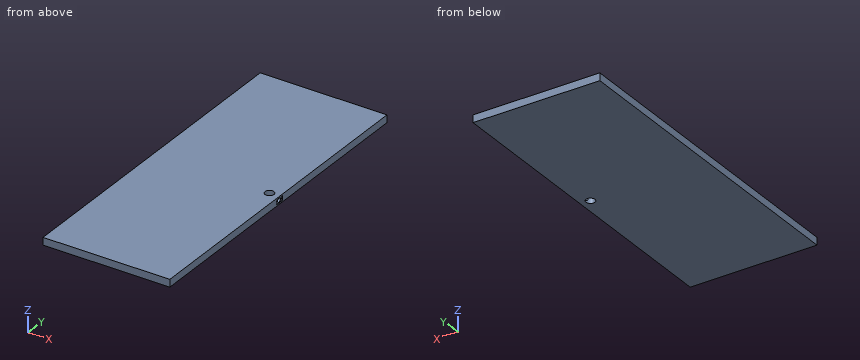
from build123d import *

# Parameters (mm, degrees)
SKETCH1_W           = 765
SKETCH1_H           = 1981
BOSS_EXTRUDE1_DEPTH = 45
SKETCH2_R           = 27
CUT_EXTRUDE1_DEPTH  = 46
CUT_EXTRUDE2_REACH  = 767
SKETCH3_R           = 12.5
SKETCH4_W           = 28.5
SKETCH4_H           = 57
CUT_EXTRUDE3_DEPTH  = 3
SKETCH5_R           = 1.5
CUT_EXTRUDE4_DEPTH  = 15


with BuildPart() as part:
    # Sketch1 → Boss-Extrude1 (new body)
    with BuildSketch(Plane.XY):
        with Locations((382.5, 990.5)):
            Rectangle(SKETCH1_W, SKETCH1_H)
    extrude(amount=BOSS_EXTRUDE1_DEPTH)

    # Sketch2 → Cut-Extrude1 (cut, through all)
    with BuildSketch(Plane.XY.offset(45)):
        with Locations((705, 1000)):
            Circle(SKETCH2_R)
    extrude(amount=-CUT_EXTRUDE1_DEPTH, mode=Mode.SUBTRACT)

    # Sketch3 → Cut-Extrude2 (cut, up to next)
    with BuildSketch(Plane(origin=(765, 0, 0), x_dir=(0, 0, -1), z_dir=(1, 0, 0)), mode=Mode.PRIVATE) as cut_extrude2_sk1:
        with Locations((-22.5, 1000)):
            Circle(SKETCH3_R)
    cut_extrude2_tool1 = extrude(cut_extrude2_sk1.sketch, amount=-CUT_EXTRUDE2_REACH, mode=Mode.PRIVATE) & part.part
    add(cut_extrude2_tool1.solids().sort_by_distance((765, 1000, 22.5))[0], mode=Mode.SUBTRACT)

    # Sketch4 → Cut-Extrude3 (cut)
    with BuildSketch(Plane(origin=(765, 0, 0), x_dir=(0, 0, -1), z_dir=(1, 0, 0))):
        with Locations((-22.5, 1000)):
            Rectangle(SKETCH4_W, SKETCH4_H)
    extrude(amount=-CUT_EXTRUDE3_DEPTH, mode=Mode.SUBTRACT)

    # Sketch5 → Cut-Extrude4 (cut)
    with BuildSketch(Plane(origin=(762, 0, 0), x_dir=(0, 0, -1), z_dir=(1, 0, 0))):
        with Locations((-22.5, 1020.5)):
            Circle(SKETCH5_R)
        with Locations((-22.5, 979.5)):
            Circle(SKETCH5_R)
    extrude(amount=-CUT_EXTRUDE4_DEPTH, mode=Mode.SUBTRACT)


solid = part.part
Build history of the part. All positions in model axes, mm. Give positions to 0.01 mm unless a question says otherwise; leave off trailing zeros. Loops run counter-clockwise (first coordinate to the right, second up) from the corner with the lowest first, then second, coordinate; pieces in that order, holes last. Notation, with made-up numbers: (41, 22) -> (91, 22) arc R32 ccw to (91, 59) -> close; hole circle Ø2 at (49, 72). An arc over 180 degrees is marked (long way). Answer in a Markdown table with one row per item.
Item 1: Probe line 1 along Y through (x, z) = (754, 22); line 2 along Y through (x, z) = (755.25, 22.5); line 3 along Z through (x, y) = (754, 1020). List the from-to ranges inside material, lowest first. Write a range as [from, to].
Findings below:
| item | result |
|---|---|
| line 1 | y = [0, 978.09], [980.91, 987.51], [1012.49, 1019.09], [1021.91, 1981] |
| line 2 | y = [0, 978], [981, 987.5], [1012.5, 1019], [1022, 1981] |
| line 3 | z = [0, 21.09], [23.91, 45] |
Item 2: Slice it at A-A on x = 705. Write the cut outline in (y, z).
Findings below:
| item | result |
|---|---|
| outline | (0, 0) -> (973, 0) -> (973, 45) -> (0, 45) -> close; (1027, 0) -> (1981, 0) -> (1981, 45) -> (1027, 45) -> close |
Item 3: Flat gauge pins, fed straight in: P1, Ø0.9, axis at y = 1020.5, z = 22.5, coming from the +X side; P2, Ø3.5, axis at y = 979.5, z = 22, coming from the +X side; P3, Ø14, axis at y = 996, z = 25.5, coming from the +X side. Where does each tip first touch, or does it go through?
Findings below:
| item | result |
|---|---|
| P1 | stops at x = 747 |
| P2 | stops at x = 762 |
| P3 | stops at x = 680.34 |
